For this review, take the finished solid that the model builds, in its own axes (mm). A direction names the side the tool comes from. Give positions to 0.01 mm unless a question says otherwise; leave off trailing zeros. Loops run counter-clockwise (first coordinate to the right, second up) from the corner with the lowest first, then second, coordinate; pieces in that order, holes last. Notation, with made-up numbers: (54, -4) - (68, -4) arc R19 ccw to (68, 28) - close; hole circle Ø7 at (30, -10.5). An arc over 180 degrees is marked (long way). Put each result on its own line as item: value.
from build123d import *

# Parameters (mm, degrees)
EXTRUDE_1_DEPTH     = 4
SKETCH_5_W          = 2
SKETCH_5_H          = 8
CUT_EXTRUDE_2_DEPTH = 10


with BuildPart() as part:
    # 草图1 → 凸台-拉伸1 (new body, symmetric)
    with BuildSketch(Plane(origin=(0, 0, 0), x_dir=(0, 0, -1), z_dir=(1, 0, 0))):
        with BuildLine():
            Line((-23, 1), (23, 1))
            ThreePointArc((23, 1), (24, 0), (23, -1))
            Line((23, -1), (-23, -1))
            ThreePointArc((-23, -1), (-24, 0), (-23, 1))
        make_face()
    extrude(amount=EXTRUDE_1_DEPTH, both=True)

    # 草图5 → 切除-拉伸2 (cut)
    with BuildSketch(Plane(origin=(0, 1, 0), x_dir=(1, 0, 0), z_dir=(0, 1, 0))):
        with Locations((-3, -20)):
            Rectangle(SKETCH_5_W, SKETCH_5_H)
        with Locations((3, -20)):
            Rectangle(SKETCH_5_W, SKETCH_5_H)
    extrude(amount=-CUT_EXTRUDE_2_DEPTH, mode=Mode.SUBTRACT)


solid = part.part
1) Insertion check: pin 1 Ø0.6 at (y, z) = (0, 21) entering from +X. The pin has a flat end and moves straight along its axis. Give the tip position at first contact, or say it passes through.
Geometry check:
pin 1: stops at x = 2
2) Take a section at A-A on y = 0.6. State the section outline as (x, z) points, and give its area (3 significant figures).
Geometry check:
outline: (-4, -23.8) - (4, -23.8) - (4, 16) - (2, 16) - (2, 23.8) - (-2, 23.8) - (-2, 16) - (-4, 16) - close
area: 350 mm²
3) Wall thickness on line 1 (Z direction, x = -3.25, y = 0.1); line 2 (X direction, y = -0.7, z = 16.5); line 3 (Z direction, x = -3, y = -0.75): over which ranges is each line inside the solid? List them lowest first.
Geometry check:
line 1: z = -23.99 to 16
line 2: x = -2 to 2
line 3: z = -23.66 to 16
4) For faces 1 (the face through (-2, 0, 20)), 2 (the face through (4, 0, -4)), 3 (the face through (2, 0, 20)), list the 3-axis set-ups (+Z, -Z, +X, -X, +Y, -Y) from which the entire face can be reached by the end or side of a thin tool; tool diameter is ignored.
Geometry check:
face 1: +Z, -X, +Y, -Y
face 2: +Z, -Z, +X, +Y, -Y
face 3: +Z, +X, +Y, -Y
5) Take a section at B-B on x = -3. State the section outline as (y, z) points.
Geometry check:
outline: (-1, -23) arc R1 ccw to (1, -23) - (1, 16) - (-1, 16) - close
